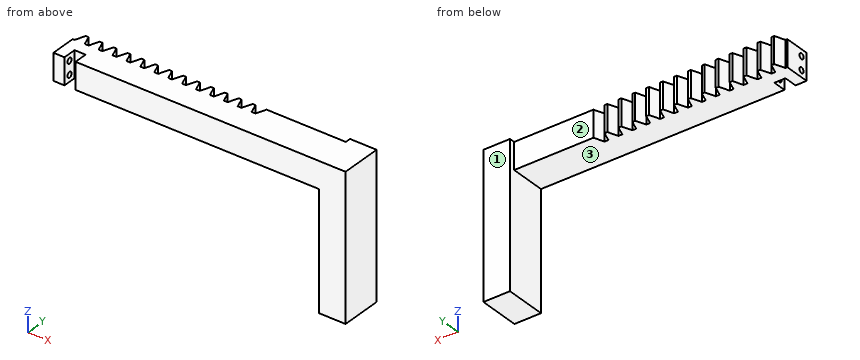
```python
from build123d import *

# Parameters (mm, degrees)
BOSS_EXTRUDE1_DEPTH = 12
SKETCH6_W           = 12
SKETCH6_H           = 11.5
BOSS_EXTRUDE4_DEPTH = 65
SKETCH7_W           = 12
SKETCH7_H           = 7
BOSS_EXTRUDE5_DEPTH = 65
SKETCH8_W           = 5
SKETCH8_H           = 6
CUT_EXTRUDE1_DEPTH  = 65
SKETCH9_W           = 34.920803936
SKETCH9_H           = 4.5
BOSS_EXTRUDE6_DEPTH = 12
SKETCH10_R          = 1.25
CUT_EXTRUDE2_DEPTH  = 12


with BuildPart() as part:
    # Sketch1 → Boss-Extrude1 (new body)
    with BuildSketch(Plane(origin=(0, 0, -6), x_dir=(-1, 0, 0), z_dir=(0, 0, -1))):
        Polygon((-70.736133614, 14.634553049), (-72.373999668, 10.134553049), (-73.855349707, 10.134553049), (-73.855349707, -1.365446951), (46.144650293, -1.365446951), (46.144650293, 10.134553049), (45.282779553, 10.134553049), (43.644913499, 14.634553049), (42.361201786, 14.634553049), (40.723335732, 10.134553049), (38.999594253, 10.134553049), (37.361728199, 14.634553049), (36.078016486, 14.634553049), (34.440150432, 10.134553049), (32.716408953, 10.134553049), (31.078542899, 14.634553049), (29.794831186, 14.634553049), (28.156965132, 10.134553049), (26.433223653, 10.134553049), (24.795357599, 14.634553049), (23.511645886, 14.634553049), (21.873779832, 10.134553049), (20.150038353, 10.134553049), (18.512172299, 14.634553049), (17.228460586, 14.634553049), (15.590594532, 10.134553049), (13.866853053, 10.134553049), (12.228986999, 14.634553049), (10.945275286, 14.634553049), (9.307409232, 10.134553049), (7.583667753, 10.134553049), (5.945801699, 14.634553049), (4.662089986, 14.634553049), (3.024223932, 10.134553049), (1.300482453, 10.134553049), (-0.337383601, 14.634553049), (-1.621095314, 14.634553049), (-3.258961368, 10.134553049), (-4.982702847, 10.134553049), (-6.620568901, 14.634553049), (-7.904280614, 14.634553049), (-9.542146668, 10.134553049), (-11.265888147, 10.134553049), (-12.903754201, 14.634553049), (-14.187465914, 14.634553049), (-15.825331968, 10.134553049), (-17.549073447, 10.134553049), (-19.186939501, 14.634553049), (-20.470651214, 14.634553049), (-22.108517268, 10.134553049), (-23.832258747, 10.134553049), (-25.470124801, 14.634553049), (-26.753836514, 14.634553049), (-28.391702568, 10.134553049), (-30.115444047, 10.134553049), (-31.753310101, 14.634553049), (-33.037021814, 14.634553049), (-34.674887868, 10.134553049), (-36.398629347, 10.134553049), (-38.036495401, 14.634553049), (-39.320207114, 14.634553049), (-40.958073168, 10.134553049), (-42.681814647, 10.134553049), (-44.319680701, 14.634553049), (-45.603392414, 14.634553049), (-47.241258468, 10.134553049), (-48.964999947, 10.134553049), (-50.602866001, 14.634553049), (-51.886577714, 14.634553049), (-53.524443768, 10.134553049), (-55.248185247, 10.134553049), (-56.886051301, 14.634553049), (-58.169763014, 14.634553049), (-59.807629068, 10.134553049), (-61.531370547, 10.134553049), (-63.169236601, 14.634553049), (-64.452948314, 14.634553049), (-66.090814368, 10.134553049), (-67.814555847, 10.134553049), (-69.452421901, 14.634553049), align=None)
    extrude(amount=-BOSS_EXTRUDE1_DEPTH)

    # Sketch6 → Boss-Extrude4 (add)
    with BuildSketch(Plane.XY.offset(6)):
        with Locations((79.855349707, 4.384553049)):
            Rectangle(SKETCH6_W, SKETCH6_H)
    extrude(amount=-BOSS_EXTRUDE4_DEPTH)

    # Sketch7 → Boss-Extrude5 (add)
    with BuildSketch(Plane.XY.offset(6)):
        with Locations((79.855349707, 13.634553049)):
            Rectangle(SKETCH7_W, SKETCH7_H)
    extrude(amount=-BOSS_EXTRUDE5_DEPTH)

    # Sketch8 → Cut-Extrude1 (cut)
    with BuildSketch(Plane.XY.offset(6)):
        with Locations((-38.644650293, 1.634553049)):
            Rectangle(SKETCH8_W, SKETCH8_H)
    extrude(amount=-CUT_EXTRUDE1_DEPTH, mode=Mode.SUBTRACT)

    # Sketch9 → Boss-Extrude6 (add)
    with BuildSketch(Plane.XY.offset(6)):
        with Locations((56.394947739, 12.384553049)):
            Rectangle(SKETCH9_W, SKETCH9_H)
    extrude(amount=-BOSS_EXTRUDE6_DEPTH)

    # Sketch10 → Cut-Extrude2 (cut)
    with BuildSketch(Plane.ZY.offset(46.144650293)):
        with Locations((-3, 1.634553049)):
            Circle(SKETCH10_R)
        with Locations((3, 1.634553049)):
            Circle(SKETCH10_R)
    extrude(amount=-CUT_EXTRUDE2_DEPTH, mode=Mode.SUBTRACT)


solid = part.part
```
Verification items for the finished model (mm, model axes). Face numbers are marked on the shaded views. A direction names the side the tool comes from. Round coordinates to 2 decimals unless told otherwise and drop trailing zeros. Order: outer loops, then holes, each group sorted by start corner. A loop starts at its lowest first (then second) coordinate and runs counter-clockwise, first axis right, second up. Notation, with made-up numbers: (18, -29.75) - (65, -29.75) arc R6 cw to (65, -23.75) - close; hole circle Ø5 at (71.25, 88). An arc over 180 degrees is marked (long way). Use CSV: the item, a comma, the result in double quotes. Start each with the question number.
1) Section check A-A, the plane x = 62.5. Record the cut outline in (y, z), plus the area to 3 significant figures.
2) Thickness scan on L1, parallel to Y at x = -42.45, z = 3; L2, parallel to Z at x = -15.5, y = 4; L3, parallel to X at y = 7.75, z = -54. Record the ranges inside material, lowest first.
3) Section check C-C, the plane y = 12.75. State how many separate pieces and enclosed holes the cut face has, plus the area to 3 significant figures.
4) Access from +Z, -Z, +X, -X, +Y, -Y to the whole of each face (thin tool, end or side, straight path). Record for the marked faces 1, 2 and 3.
5) Go/stop test with flat-tipped pins: P1, Ø2, axis at x = 41, z = -1, coming from the +Y side; P2, Ø5, axis at x = 16, y = 5, coming from the -Z side; P3, Ø0.9, axis at x = -27.5, z = 1.5, coming from the +Y side; P4, Ø5, axis at y = 1.5, z = 2.5, coming from the -X side. Record where each tip stops, or that it passes through.
6) Section check B-B, the plane z = -45.5. Record the cut outline in (x, y), plus the area to 3 significant figures.
Answers:
1,outline,"(-1.37, -6) - (14.63, -6) - (14.63, 6) - (-1.37, 6) - close"
1,area,"192 mm²"
2,L1,"y = -1.37 to 0.38, 2.88 to 14.63"
2,L2,"z = -6 to 6"
2,L3,"x = 73.86 to 85.86"
3,separate pieces,"14"
3,enclosed holes,"0"
3,area,"1,630 mm²"
4,face 1,"+Z, -Z, +X, -X, +Y"
4,face 2,"+Z, -Z, -X, +Y"
4,face 3,"-Z, -X, +Y, -Y"
5,P1,"stops at y = 14.63"
5,P2,"stops at z = -6"
5,P3,"stops at y = 10.13"
5,P4,"stops at x = -46.14"
6,outline,"(73.86, -1.37) - (85.86, -1.37) - (85.86, 17.13) - (73.86, 17.13) - close"
6,area,"222 mm²"
